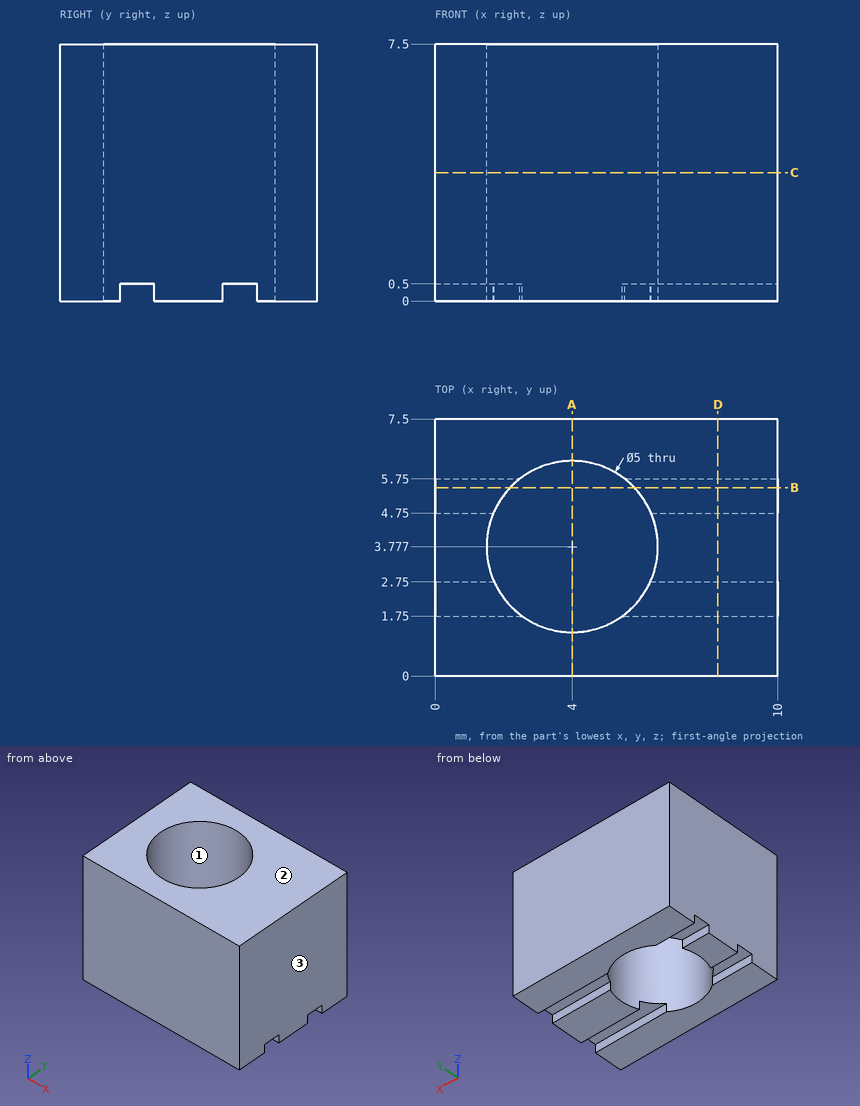
Design review of the part shown in the three views and the two pictorial views. Dimensions are in mm from the part's minimum x, y and z. Give positions to 0.01 mm unless a question says otherwise; leave off trailing zeros. Loops run counter-clockwise (first coordinate to the right, second up) from the corner with the lowest first, then second, coordinate; pieces in that order, holes last. Notation, with made-up numbers: (69, -29) -> (110, -29) arc R35 ccw to (110, 4) -> close; hole circle Ø5 at (-3.5, 34.25). An arc over 180 degrees is marked (long way). Put each result on its own line as item: value. Start each with the question number.
1. Mouldability with a two-part tool opening along X and no side actions: class the marked faces 1, 2 and 3 as released by +X, released by -X, zero draft, split by the parting line, or undercut.
2. We need section C-C on z = 3.75. State the section outline as (x, y) points.
3. We need section B-B on y = 5.5. State the section outline as (x, z) points.
4. We need section A-A on x = 4. State the section outline as (y, z) points.
5. We need section D-D on x = 8.25. State the section outline as (y, z) points.
6. Clearance check with a flat-ended pin moving along its axis: P1, Ø4.5, axis at x = 4, y = 3.78, coming from the -Z side. State where the tip first meets the part, or that it passes through.
7. Wall thickness on probe 1 along Y at (x, z) = (4, 2.5); probe 2 along X at (y, z) = (1.75, 5.25) (1 decimal); probe 3 along Y at (x, z) = (2.75, 1.25): over which ranges is each line inside the solid? List them lowest first.
Determined:
1. face 1: undercut
1. face 2: zero draft
1. face 3: released by +X
2. outline: (0, 0) -> (10, 0) -> (10, 7.5) -> (0, 7.5) -> close; hole circle Ø5 at (4, 3.78)
3. outline: (0, 0.5) -> (2.19, 0.5) -> (2.19, 7.5) -> (0, 7.5) -> close; (5.81, 0.5) -> (10, 0.5) -> (10, 7.5) -> (5.81, 7.5) -> close
4. outline: (0, 0) -> (1.28, 0) -> (1.28, 7.5) -> (0, 7.5) -> close; (6.28, 0) -> (7.5, 0) -> (7.5, 7.5) -> (6.28, 7.5) -> close
5. outline: (0, 0) -> (1.75, 0) -> (1.75, 0.5) -> (2.75, 0.5) -> (2.75, 0) -> (4.75, 0) -> (4.75, 0.5) -> (5.75, 0.5) -> (5.75, 0) -> (7.5, 0) -> (7.5, 7.5) -> (0, 7.5) -> close
6. P1: through
7. probe 1: 0 to 1.28, 6.28 to 7.5
7. probe 2: 0 to 2.5, 5.5 to 10
7. probe 3: 0 to 1.61, 5.94 to 7.5
